Verification items for the finished model (mm, model axes). Face numbers are marked on the shaded views. Round coordinates to 2 decimals unless told otherwise and drop trailing zeros. Write each loop counter-clockwise with the first axis right and the second up, starting at its lowest first coordinate (ties: lowest second). Pieces come first, ordered by that corner, then holes. Notation, with made-up numbers: M 19,48 L 38,48 A11 cw 38,60 Z; hole C 64.5,-0.5 d11. An arc over 180 degrees is marked long. Answer in a Markdown table with one row per item. Add a question column.
1. Material ranges on probe 1 along Z at (x, y) = (0, 41); probe 2 along Y at (x, z) = (-43, 0); probe 3 along X at (y, z) = (56, -1.5) (3 decimals), recorded low to high.
2. Draft check along X on the marked faces 1, 2 and 3. Enter one of: pulls with the +X half, pulls with the -X half, needs draft (parallel to the pull), parting line crosses it, or undercut.
3. Sectioned sample at B-B on z = 0. Record the cut outline in (x, y).
4. Sectioned sample at C-C on y = 55.5. Record the cut outline in (x, z).
5. Sectioned sample at D-D on z = -26. Record the cut outline in (x, y).
6. Go/stop test with flat-tipped pins: pin 1 Ø12 at (x, y) = (-55.5, 53) entering from -Z; pin 2 Ø12 at (y, z) = (23, -0.5) entering from -X; pin 3 Ø16 at (y, z) = (6, -68) entering from +X. Record where each tip stops, or that it passes through.
7. Sectioned sample at A-A on x = 0. Record the cut outline in (y, z), plus the area to 3 significant figures.
```python
from build123d import *

# Parameters (mm, degrees)
SKETCH2_R               = 45
SKETCH2_R_2             = 42.5
BOSS_EXTRUDE1_DEPTH     = 60
CUT_EXTRUDE1_DEPTH      = 88.464278423
CUT_EXTRUDE1_DEPTH_BACK = 88.464278423
CUT_EXTRUDE2_DEPTH      = 88.464278423
CUT_EXTRUDE2_DEPTH_BACK = 88.464278423
SKETCH4_R               = 5
BOSS_EXTRUDE2_DEPTH     = 20
MIRROR1_DEPTH           = 20


# Read off the part's stored shape, not the designer's step: Mirror1
with BuildPart() as part:
    # Sketch2 → Boss-Extrude1 (new body)
    with BuildSketch(Plane(origin=(0, 0, 0), x_dir=(1, 0, 0), z_dir=(0, 1, 0))):
        with Locations(Location((0, 0, 0), (0, 0, 270))):
            Circle(SKETCH2_R)
        with Locations(Location((0, 0, 0), (0, 0, 270))):
            Circle(SKETCH2_R_2, mode=Mode.SUBTRACT)
    extrude(amount=BOSS_EXTRUDE1_DEPTH)

    # Sketch3 → Cut-Extrude1 (cut, two sides: drawn at the far end of the back side and taken through both)
    with BuildSketch(Plane.XY.offset(-CUT_EXTRUDE1_DEPTH_BACK)):
        Polygon((-30, 0), (45, 40), (45, 0), align=None)
    extrude(amount=CUT_EXTRUDE1_DEPTH + CUT_EXTRUDE1_DEPTH_BACK, mode=Mode.SUBTRACT)

    # Sketch4 → Cut-Extrude2 (cut, two sides: drawn at the far end of the back side and taken through both)
    with BuildSketch(Plane(origin=(0, 0, 0), x_dir=(0, 0, -1), z_dir=(1, 0, 0)).offset(-CUT_EXTRUDE2_DEPTH_BACK)):
        with Locations((0, 15)):
            Circle(SKETCH4_R)
    extrude(amount=CUT_EXTRUDE2_DEPTH + CUT_EXTRUDE2_DEPTH_BACK, mode=Mode.SUBTRACT)

    # Sketch5 → Boss-Extrude2 (add)
    with BuildSketch(Plane(origin=(0, 0, 0), x_dir=(1, 0, 0), z_dir=(0, 1, 0))):
        with BuildLine():
            ThreePointArc((-22.426406871, 39.013539635), (-34.577946498, 28.798708582), (-42.426406871, 15))
            ThreePointArc((-42.426406871, 15), (-100.617737833, -6.538529057), (-162.426406871, -12))
            Line((-162.426406871, -12), (-162.426406871, 69.013539635))
            Line((-162.426406871, 69.013539635), (-22.426406871, 69.013539635))
            Line((-22.426406871, 69.013539635), (-22.426406871, 39.013539635))
        make_face()
    extrude(amount=BOSS_EXTRUDE2_DEPTH)

    # Mirror1 outline → Mirror1 (add)
    with BuildSketch(Plane(origin=(0, 0, 0), x_dir=(1, 0, 0), z_dir=(0, 1, 0))):
        with BuildLine():
            Line((-22.426406871, 69.013539635), (-22.426406871, 99.013539635))
            ThreePointArc((-22.426406871, 99.013539635), (-34.577946498, 109.228370688), (-42.426406871, 123.02707927))
            ThreePointArc((-42.426406871, 123.02707927), (-100.617737833, 144.565608327), (-162.426406871, 150.02707927))
            Line((-162.426406871, 150.02707927), (-162.426406871, 69.013539635))
            Line((-162.426406871, 69.013539635), (-22.426406871, 69.013539635))
        make_face()
    extrude(amount=MIRROR1_DEPTH)


solid = part.part
```
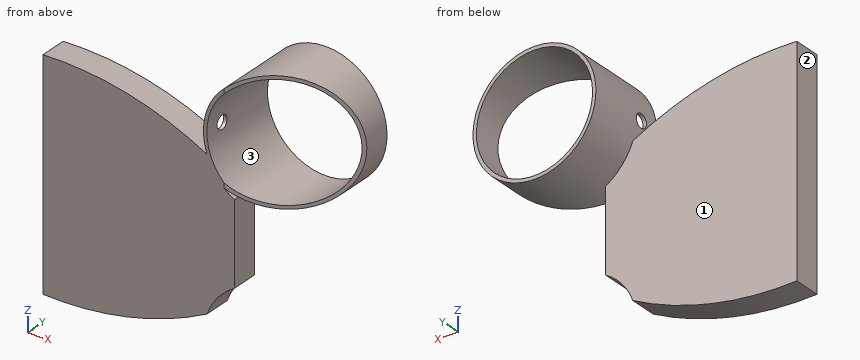
Geometry check:
| question | item | result |
|---|---|---|
| 1 | probe 1 | z = -45 to -42.5, 42.5 to 45 |
| 1 | probe 2 | y = 0 to 10, 20 to 60 |
| 1 | probe 3 | x = -44.975 to -42.474, 42.474 to 44.975 |
| 2 | face 1 | needs draft |
| 2 | face 2 | pulls with the -X half |
| 2 | face 3 | undercut |
| 3 | outline | M -162.43,0 L -77.28,0 L -77.28,20 L -162.43,20 Z; M -45,0 L -42.5,0 L -42.5,10 L -45,10 Z; M -45,20 L -42.5,20 L -42.5,60 L -45,60 Z; M 42.5,38.67 L 45,40 L 45,60 L 42.5,60 Z |
| 4 | outline | C 0,0 d90; hole C 0,0 d85 |
| 5 | outline | M -162.43,0 L -33.62,0 L -33.62,60 L -36.73,60 L -36.73,20 L -162.43,20 Z; M 33.62,33.93 L 36.73,35.59 L 36.73,60 L 33.62,60 Z |
| 6 | pin 1 | passes through |
| 6 | pin 2 | stops at x = -162.43 |
| 6 | pin 3 | stops at x = -22.43 |
| 7 | outline | M 16,-45 L 60,-45 L 60,-42.5 L 16,-42.5 Z; M 16,42.5 L 60,42.5 L 60,45 L 16,45 Z |
| 7 | area | 220 mm2 |
